For this review, take the finished solid that the model builds, in its own axes (mm). Face numbers are marked on the shaded views. A direction names the side the tool comes from. Give positions to 0.01 mm unless a question says otherwise; leave off trailing zeros. Write each loop counter-clockwise with the first axis right and the second up, starting at its lowest first coordinate (ties: lowest second). Pieces come first, ordered by that corner, then holes. Notation, with made-up numbers: M 88.25,52 L 102.25,52 A24 cw 102.25,68 Z; hole C 5.25,28.25 d5. An arc over 180 degrees is marked long. Answer as a JSON object with one key per item and string values. Group by question number.
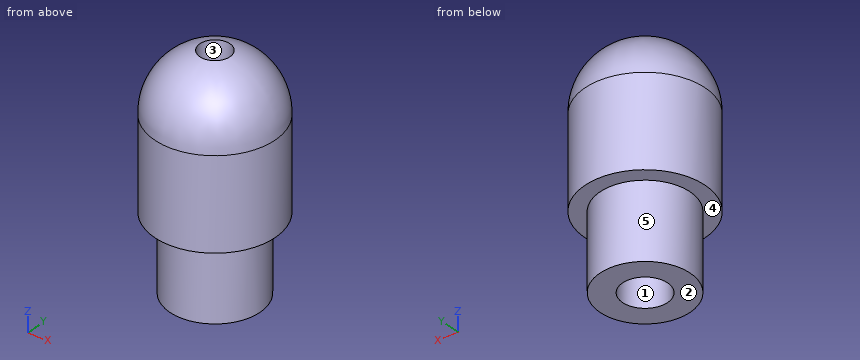
```python
from build123d import *


with BuildPart() as part:
    # Sketch → Revolution (revolve)
    with BuildSketch(Plane(origin=(0, 0, 300), x_dir=(0, 0, -1), z_dir=(1, 0, 0))):
        with BuildLine():
            Line((0, 4), (6, 4))
            Line((6, 4), (6, 3))
            Line((6, 3), (11, 3))
            Line((11, 3), (11, 1.5))
            Line((11, 1.5), (8, 1.5))
            Line((8, 1.5), (8, 1))
            Line((8, 1), (-3.925111, 1))
            ThreePointArc((0, 4), (-2.481046, 3.178377), (-3.925111, 1))
        make_face()
    revolve(axis=Axis((0, 0, 300), (0, 0, -1)))


solid = part.part
```
Item 1: Machinability: for the marked faces 1 and 2, which of the approach directions +Z, -Z, +X, -X, +Y, -Y give a long, thin tool a straight path to every point of the face, cutting with its end or side? Answer none if there is none.
Item 2: Insertion check: P1, Ø3, axis at x = 0, y = 0, coming from the +Z side; P2, Ø1, axis at y = 1, z = 302, coming from the +X side. Each pin has a flat end and moves straight along its axis. Give the tip position at first contact, or say it passes through.
Item 3: To check wall thickness, follow probe 1 along X at (y, z) = (0, 294.5); probe 2 along X at (y, z) = (1, 291.5); probe 3 along Y at (x, z) = (0.5, 292.75). State the ranges of each line that lie inside material, in increasing order.
Item 4: Draft analysis for pull direction Y (two halves, no side actions). For the marked faces 3, 4 and 5, state which applies: released by +Y, released by -Y, zero draft, split by the parting line, or undercut.
Item 5: Consider section A-A (z = 294.75). Give the boundary of the cut face in (x, y), plus the area to 3 significant figures.
Item 6: Consider section B-B (z = 292.5). Give the boundary of the cut face in (x, y), plus the area to 3 significant figures.
Result set:
{
 "1": {"face 1": "-Z", "face 2": "-Z, +X, -X, +Y, -Y"},
 "2": {"P1": "stops at z = 303.93", "P2": "stops at x = 3.63"},
 "3": {"probe 1": "x = -4 to -1, 1 to 4", "probe 2": "x = -2.83 to -1.12, 1.12 to 2.83", "probe 3": "y = -2.96 to -0.87, 0.87 to 2.96"},
 "4": {"face 3": "undercut", "face 4": "zero draft", "face 5": "split by the parting line"},
 "5": {"outline": "C 0,0 d8; hole C 0,0 d2", "area": "47.1 mm^2"},
 "6": {"outline": "C 0,0 d6; hole C 0,0 d2", "area": "25.1 mm^2"}
}
